Build history of the part. All positions in model axes, mm. A direction names the side the tool comes from. Give positions to 0.01 mm unless a question says otherwise; leave off trailing zeros. Write each loop counter-clockwise with the first axis right and the second up, starting at its lowest first coordinate (ties: lowest second). Pieces come first, ordered by that corner, then holes.
from build123d import *

# Parameters (mm, degrees)
BOSS_EXTRUDE2_DEPTH = 4
BOSS_EXTRUDE3_DEPTH = 2
BOSS_EXTRUDE4_DEPTH = 4
SKETCH5_W           = 5.555
SKETCH5_H           = 3.214115871
CUT_EXTRUDE1_DEPTH  = 6


with BuildPart() as part:
    # Sketch2 → Boss-Extrude2 (new body)
    with BuildSketch(Plane(origin=(0, 0, 0), x_dir=(1, 0, 0), z_dir=(0, 1, 0))):
        Polygon((5.5, 6.858588715), (-7.617234461, 6.858588715), (-9.959191583, 4.257581826), (-1.338261213, -1.486289651), (42.73, -4), (49.538362829, 1.796672871), (47.61, 4.0948062), (47.61, 8.9), (16.61, 8.9), (16.61, 0), (5.5, 0), align=None)
    extrude(amount=BOSS_EXTRUDE2_DEPTH)

    # Sketch2<9> → Boss-Extrude3 (add)
    with BuildSketch(Plane(origin=(0, 0, 0), x_dir=(1, 0, 0), z_dir=(0, 1, 0))):
        with BuildLine():
            Line((-0.115159211, -0.3), (-7.817973643, 6.635645268))
            Line((-7.817973643, 6.635645268), (-9.959191583, 4.257581826))
            Line((-9.959191583, 4.257581826), (-1.338261213, -1.486289651))
            Line((-1.338261213, -1.486289651), (42.73, -4))
            Line((42.73, -4), (49.538362829, 1.796672871))
            Line((49.538362829, 1.796672871), (47.802836283, 3.864992867))
            Line((47.802836283, 3.864992867), (42.83919107, -0.3))
            Line((42.83919107, -0.3), (34.16881591, -0.3))
            Line((34.16881591, -0.3), (34.16881591, 0.607570661))
            ThreePointArc((34.16881591, 0.607570661), (29.26, 4.2), (24.35118409, 0.607570661))
            Line((24.35118409, 0.607570661), (24.35118409, -0.3))
            Line((24.35118409, -0.3), (-0.115159211, -0.3))
        make_face()
    extrude(amount=-BOSS_EXTRUDE3_DEPTH)

    # Sketch4 → Boss-Extrude4 (add)
    with BuildSketch(Plane(origin=(0, -2, 0), x_dir=(-1, 0, 0), z_dir=(0, -1, 0))):
        Polygon((-47.61, 8.9), (-47.61, 4.0948062), (-49.538362829, 1.796672871), (-42.73, -4), (1.338261213, -1.486289651), (9.959191583, 4.257581826), (7.617234461, 6.858588715), (0, 6.858588715), (0, 0), (-24.15118409, 0), (-24.15118409, 8.9), align=None)
    extrude(amount=BOSS_EXTRUDE4_DEPTH)

    # Sketch5 → Cut-Extrude1 (cut)
    with BuildSketch(Plane(origin=(0, -6, 0), x_dir=(-1, 0, 0), z_dir=(0, -1, 0))):
        Polygon((-25.659003688, 8.9), (-23.590958237, 8.9), (-23.590958237, 0), (-24.15118409, 0), align=None)
        Polygon((-23.590958237, 0), (-16.61, -3.214115871), (-16.61, 0), align=None)
        with Locations((-13.8325, -1.607057936)):
            Rectangle(SKETCH5_W, SKETCH5_H)
        with Locations((-8.2775, -1.607057936)):
            Rectangle(SKETCH5_W, SKETCH5_H)
        Polygon((-5.5, -3.214115871), (-0.689386067, 0), (-5.5, 0), align=None)
        Polygon((0, 0), (-0.689386067, 0), (-0.689386067, 6.858588715), (0, 6.858588715), (1.904308615, 6.858588715), align=None)
    extrude(amount=-CUT_EXTRUDE1_DEPTH, mode=Mode.SUBTRACT)


solid = part.part
(1) Saw through at C-C, the plane y = 2.25. List the corners of the cut face in (x, z), plus the area to 3 significant figures.
(2) Saw through at D-D, the plane x = 43.5. List the corners of the cut face in (y, z), plus the area to 3 significant figures.
(3) Drop flat-ended pins along their axis: pin 1 (0.6 mm diameter, centred on x = 0.5, y = -1, fed in from -Z); pin 2 (4.5 mm diameter, centred on x = 1, y = 2.5, fed in from -Z); pin 3 (1.2 mm diameter, centred on y = 3, z = -7, fed in from +X). Give the stop position or say it passes through.
(4) Probe line 1 (Y direction, x = 35, z = -6.75); line 2 (Y direction, x = 19, z = -5.25); line 3 (X direction, y = -0.25, z = -2.75). List the from-to ranges inside material, lowest first.
(5) Saw through at B-B, the plane y = -3.5. List the corners of the cut face in (x, z).
(6) Mould opens along X. For faces 4 (the face through (20.82, -3.042, 1.276)), 5 (the face through (-1, 2, -6.859)), 6 (the face through (47.61, -4, -7)) say: +X half, -X half, draft (parallel to the pull), parting line (faces both ways), or undercut.
(7) 3-axis set-ups, long thin cutter, end or side, ignore diameter. For faces 1 (the face through (24, -1, 0.3)), 2 (the face through (5.5, 2, -3)), 3 (the face through (47.61, 2, -6)): which of +Z, -Z, +X, -X, +Y, -Y reach the whole face in a straight line?
(8) Saw through at A-A, the plane z = -2.5. List the corners of the cut face in (x, y).
Computed values:
1. outline: (-9.96, -4.26) - (-7.62, -6.86) - (5.5, -6.86) - (5.5, 0) - (16.61, 0) - (16.61, -8.9) - (47.61, -8.9) - (47.61, -4.09) - (49.54, -1.8) - (42.73, 4) - (-1.34, 1.49) - close
1. area: 501 mm2
2. outline: (-6, -8.9) - (-2, -8.9) - (-2, -0.25) - (0, -0.25) - (0, -8.9) - (4, -8.9) - (4, 3.34) - (-6, 3.34) - close
2. area: 105 mm2
3. pin 1: stops at z = 0.3
3. pin 2: stops at z = -6.86
3. pin 3: stops at x = 47.61
4. line 1: y = -6 to -2, 0 to 4
4. line 2: y = 0 to 4
4. line 3: x = -7.7 to -3.5, 25.68 to 32.84, 46.47 to 48.74
5. outline: (-9.96, -4.26) - (-7.62, -6.86) - (-1.9, -6.86) - (0, 0) - (0.69, 0) - (3.31, 1.75) - (-1.34, 1.49) - close; (17.97, 2.59) - (23.59, 0) - (24.15, 0) - (25.66, -8.9) - (47.61, -8.9) - (47.61, -4.09) - (49.54, -1.8) - (42.73, 4) - close
6. face 4: undercut
6. face 5: draft
6. face 6: +X half
7. face 1: -Z
7. face 2: -Z, +Y, -Y
7. face 3: -Z, +X, +Y, -Y
8. outline: (-7.32, -6) - (-0.69, -6) - (-0.69, -2) - (-3.22, -2) - (-3.22, 0) - (5.5, 0) - (5.5, 4) - (-7.32, 4) - close; (16.61, 0) - (25.44, 0) - (25.44, -2) - (24.57, -2) - (24.57, -6) - (48.95, -6) - (48.95, 4) - (16.61, 4) - close; hole (33.08, -2) - (46.18, -2) - (46.18, 0) - (33.08, 0) - close
